from build123d import *

# Parameters (mm, degrees)
SKETCH_1_W          = 93
SKETCH_1_H          = 64
EXTRUDE_1_DEPTH     = 2
SKETCH_3_W          = 78
SKETCH_3_H          = 51
EXTRUDE_2_DEPTH     = 8
SKETCH_4_R          = 1.5
CUT_EXTRUDE_1_DEPTH = 114.176852757
SKETCH_5_W          = 68
SKETCH_5_H          = 41
CUT_EXTRUDE_2_DEPTH = 0.5
SKETCH_6_R          = 0.5
EXTRUDE_3_DEPTH     = 10


with BuildPart() as part:
    # 草图1 → 凸台-拉伸1 (new body)
    with BuildSketch(Plane.XY):
        with Locations((46.5, 32)):
            Rectangle(SKETCH_1_W, SKETCH_1_H)
    extrude(amount=EXTRUDE_1_DEPTH)

    # 草图3 → 凸台-拉伸2 (add)
    with BuildSketch(Plane.XY.offset(2)):
        with Locations((46.5, 32)):
            Rectangle(SKETCH_3_W, SKETCH_3_H)
    extrude(amount=EXTRUDE_2_DEPTH)

    # 草图4 → 切除-拉伸1 (cut, through all)
    with BuildSketch(Plane.XY.offset(2)):
        with Locations((2.5, 61.5)):
            Circle(SKETCH_4_R)
        with Locations(Location((90.5, 61.5, 0), (0, 0, 180))):
            Circle(SKETCH_4_R)
        with Locations((90.5, 2.5)):
            Circle(SKETCH_4_R)
        with Locations(Location((2.5, 2.5, 0), (0, 0, 180))):
            Circle(SKETCH_4_R)
    extrude(amount=-CUT_EXTRUDE_1_DEPTH, mode=Mode.SUBTRACT)

    # 草图5 → 切除-拉伸2 (cut)
    with BuildSketch(Plane.XY.offset(10)):
        with Locations((46.5, 32)):
            Rectangle(SKETCH_5_W, SKETCH_5_H)
    extrude(amount=-CUT_EXTRUDE_2_DEPTH, mode=Mode.SUBTRACT)

    # 草图6 → 凸台-拉伸3 (add)
    with BuildSketch(Plane.XY.offset(2)):
        with Locations((14, 2)):
            Circle(SKETCH_6_R)
        with Locations((16.54, 2)):
            Circle(SKETCH_6_R)
        with Locations((19.08, 2)):
            Circle(SKETCH_6_R)
        with Locations((21.62, 2)):
            Circle(SKETCH_6_R)
        with Locations((24.16, 2)):
            Circle(SKETCH_6_R)
        with Locations((26.7, 2)):
            Circle(SKETCH_6_R)
        with Locations((29.24, 2)):
            Circle(SKETCH_6_R)
        with Locations((31.78, 2)):
            Circle(SKETCH_6_R)
        with Locations((34.32, 2)):
            Circle(SKETCH_6_R)
        with Locations((36.86, 2)):
            Circle(SKETCH_6_R)
        with Locations((39.4, 2)):
            Circle(SKETCH_6_R)
        with Locations((41.94, 2)):
            Circle(SKETCH_6_R)
        with Locations((44.48, 2)):
            Circle(SKETCH_6_R)
        with Locations((47.02, 2)):
            Circle(SKETCH_6_R)
        with Locations((49.56, 2)):
            Circle(SKETCH_6_R)
        with Locations((52.1, 2)):
            Circle(SKETCH_6_R)
        with Locations((54.64, 2)):
            Circle(SKETCH_6_R)
        with Locations((57.18, 2)):
            Circle(SKETCH_6_R)
        with Locations((59.72, 2)):
            Circle(SKETCH_6_R)
        with Locations((62.26, 2)):
            Circle(SKETCH_6_R)
    extrude(amount=-EXTRUDE_3_DEPTH)


solid = part.part
Geometry: final body of the model. Coordinates: model frame, mm. A direction names the side the tool comes from. Round coordinates to 2 decimals unless told otherwise and drop trailing zeros. Loops run counter-clockwise (first coordinate to the right, second up) from the corner with the lowest first, then second, coordinate; pieces in that order, holes last.
Q1. Pull-direction query (X, two-part tool) for faces 4 (the flat face through (46, 32, 9.5)), 5 (the cylindrical face through (2.305, 62.987, 1.014)), 6 (the flat face through (0, 32, 1)), 7 (the flat face through (46, 64, 1)); classes: released by +X, released by -X, zero draft, split by the parting line, or undercut.
Q2. Section A-A on z = -1.5. State how many separate pieces and enclosed holes the cut face has, plus the area to 3 significant figures.
Q3. Pin query (flat end, axial travel): P1, Ø3, axis at y = 11.5, z = 4, coming from the -X side; P2, Ø3, axis at x = 55, z = -2, coming from the -Y side; P3, Ø19, axis at x = 43, y = 39.5, coming from the +Z side; P4, Ø1.8, axis at x = 90.5, y = 2.5, coming from the -Z side. Return the tip coordinate at first contact, or that it passes through.
Q4. Access query for faces 1 (the flat face through (85.5, 32, 6)), 2 (the flat face through (7.5, 32, 6)), 3 (the flat face through (46, 6.5, 6)). Directions: +Z, -Z, +X, -X, +Y, -Y. A direction counts if a zero-diameter tool reaches every point of the face in a straight line with its end or side. Return the directions, or none.
Q5. Section C-C on x = 2.5. Return loops of the section in (y, z).
Q6. Section B-B on y = 61.5. Return loops of the section in (x, z).
Q7. Material intervals for L1, parallel to Y at x = 90.5, z = 0.95; L2, parallel to Z at x = 11.5, y = 5; L3, parallel to Z at x = 16.5, y = 36, sorted ascending.
Q8. Section D-D on y = 28. Return loops of the section in (x, z), plus the area to 3 significant figures.
Evaluation:
1. face 4: undercut
1. face 5: undercut
1. face 6: released by -X
1. face 7: zero draft
2. separate pieces: 20
2. enclosed holes: 0
2. area: 15.7 mm2
3. P1: stops at x = 7.5
3. P2: stops at y = 1.5
3. P3: stops at z = 9.5
3. P4: passes through
4. face 1: +Z, +X, +Y, -Y
4. face 2: +Z, -X, +Y, -Y
4. face 3: +Z, +X, -X, -Y
5. outline: (0, 0) - (1, 0) - (1, 2) - (0, 2) - close; (4, 0) - (60, 0) - (60, 2) - (4, 2) - close; (63, 0) - (64, 0) - (64, 2) - (63, 2) - close
6. outline: (0, 0) - (1, 0) - (1, 2) - (0, 2) - close; (4, 0) - (89, 0) - (89, 2) - (4, 2) - close; (92, 0) - (93, 0) - (93, 2) - (92, 2) - close
7. L1: y = 0 to 1, 4 to 60, 63 to 64
7. L2: z = 0 to 2
7. L3: z = 0 to 9.5
8. outline: (0, 0) - (93, 0) - (93, 2) - (85.5, 2) - (85.5, 10) - (80.5, 10) - (80.5, 9.5) - (12.5, 9.5) - (12.5, 10) - (7.5, 10) - (7.5, 2) - (0, 2) - close
8. area: 776 mm2
